Model file for the job. Use its own axes, mm. A direction names the side the tool comes from. Round coordinates to 2 decimals unless told otherwise and drop trailing zeros. Loops run counter-clockwise (first coordinate to the right, second up) from the corner with the lowest first, then second, coordinate; pieces in that order, holes last. Notation, with made-up numbers: (80, -38.75) - (119, -38.75) arc R21 ccw to (119, -14.75) - close; hole circle Ø6 at (20.25, 56). An arc over 180 degrees is marked (long way). Answer as a JSON object with one key per item and string values.
from build123d import *

# Parameters (mm, degrees)
SZKIC1_R                    = 7.5
SZKIC1_R_2                  = 5
DODANIE_WYCI_GNI_CIE1_DEPTH = 40
DODANIE_WYCI_GNI_CIE2_START = 10
SZKIC1_2_R                  = 5
DODANIE_WYCI_GNI_CIE2_DEPTH = 50
SZKIC2_OUTSIDE_W            = 29.728
SZKIC2_OUTSIDE_H            = 29.728
SZKIC2_OUTSIDE_W_2          = 10
SZKIC2_OUTSIDE_H_2          = 7
WYTNIJ_WYCI_GNI_CIE1_DEPTH  = 18
SZKIC3_R                    = 1.5
WYTNIJ_WYCI_GNI_CIE2_DEPTH  = 10


with BuildPart() as part:
    # Szkic1 → Dodanie-wyci_gni_cie1 (new body)
    with BuildSketch(Plane(origin=(0, 0, 0), x_dir=(1, 0, 0), z_dir=(0, 1, 0))):
        Circle(SZKIC1_R)
        Circle(SZKIC1_R_2, mode=Mode.SUBTRACT)
    extrude(amount=DODANIE_WYCI_GNI_CIE1_DEPTH)

    # Szkic1_2 → Dodanie-wyci_gni_cie2 (add)
    with BuildSketch(Plane(origin=(0, 0, 0), x_dir=(1, 0, 0), z_dir=(0, 1, 0)).offset(DODANIE_WYCI_GNI_CIE2_START)):
        Circle(SZKIC1_2_R)
    extrude(amount=DODANIE_WYCI_GNI_CIE2_DEPTH)

    # Szkic2 outside → Wytnij-wyci_gni_cie1 (cut)
    with BuildSketch(Plane(origin=(0, 60, 0), x_dir=(1, 0, 0), z_dir=(0, 1, 0))):
        Rectangle(SZKIC2_OUTSIDE_W, SZKIC2_OUTSIDE_H)
        Rectangle(SZKIC2_OUTSIDE_W_2, SZKIC2_OUTSIDE_H_2, mode=Mode.SUBTRACT)
    extrude(amount=-WYTNIJ_WYCI_GNI_CIE1_DEPTH, mode=Mode.SUBTRACT)

    # Szkic3 → Wytnij-wyci_gni_cie2 (cut)
    with BuildSketch(Plane.XY.offset(3.5)):
        with Locations((0, 57)):
            Circle(SZKIC3_R)
    extrude(amount=-WYTNIJ_WYCI_GNI_CIE2_DEPTH, mode=Mode.SUBTRACT)


solid = part.part
1) Two-plate mould, pull along Z, no slides. Class faces 5 (the flat face through (0, 10, 0)), 6 (the flat face through (2, 0, 5)), 7 (the flat face through (0, 51, -3.5)), 8 (the cylindrical face through (-1.08, 4.93, 4.88)): pulls with the +Z half, pulls with the -Z half, needs draft (parallel to the pull), parting line crosses it, or undercut.
Values follow:
{"face 5": "undercut", "face 6": "needs draft", "face 7": "pulls with the -Z half", "face 8": "undercut"}
2) Drop flat-ended pins along their axis: P1, Ø3, axis at x = -4.5, y = 53, coming from the +Z side; P2, Ø4, axis at x = 4, y = 28.5, coming from the +Z side; P3, Ø0.8, axis at x = 0.5, z = -4, coming from the +Y side. Give the stop position or say it passes through.
Values follow:
{"P1": "z = 3.5", "P2": "z = 7.23", "P3": "y = 42"}
3) Probe probe 1 along X at (y, z) = (2.5, 0); probe 2 along Y at (x, z) = (-4, 3.5). List the from-to ranges inside material, lowest first.
Values follow:
{"probe 1": "-7.5 to -5, 5 to 7.5", "probe 2": "0 to 40"}
4) Slice it at C-C on z = 0. List the corners of the cut face in (x, y).
Values follow:
{"outline": "(-7.5, 0) - (-5, 0) - (-5, 10) - (5, 10) - (5, 0) - (7.5, 0) - (7.5, 40) - (5, 40) - (5, 60) - (-5, 60) - (-5, 40) - (-7.5, 40) - close; hole circle Ø3 at (0, 57)"}
5) Slice it at D-D on y = 4. List the corners of the cut face in (x, z).
Values follow:
{"outline": "circle Ø15 at (0, 0); hole circle Ø10 at (0, 0)"}
6) Slice it at A-A on y = 57. List the corners of the cut face in (x, z), then the cut area to 3 significant figures.
Values follow:
{"outline": "(-3.57, -3.5) - (-1.5, -3.5) - (-1.5, 3.5) - (-3.57, 3.5) arc R5 ccw to start; (1.5, -3.5) - (3.57, -3.5) arc R5 ccw to (3.57, 3.5) - (1.5, 3.5) - close", "area": "42.8 mm²"}
7) Slice it at B-B on x = 0. List the corners of the cut face in (y, z), then the cut area to 3 significant figures.
Values follow:
{"outline": "(0, -7.5) - (40, -7.5) - (40, -5) - (42, -5) - (42, -3.5) - (55.5, -3.5) - (55.5, 3.5) - (42, 3.5) - (42, 5) - (40, 5) - (40, 7.5) - (0, 7.5) - (0, 5) - (10, 5) - (10, -5) - (0, -5) - close; (58.5, -3.5) - (60, -3.5) - (60, 3.5) - (58.5, 3.5) - close", "area": "625 mm²"}
8) Tool access for faces 1 (the cylindrical face through (-5, 50, 0)), 2 (the cylindrical face through (-0.195, 58.487, 0.049)), 3 (the flat face through (0, 51, 3.5)), 4 (the flat face through (0, 42, -4)): list every direction of +Z, -Z, +X, -X, +Y, -Y with a clear straight run to the whole face (end or side of a thin tool).
Values follow:
{"face 1": "+Y", "face 2": "+Z, -Z", "face 3": "+Z, +X, -X, +Y", "face 4": "-Z, +X, -X, +Y"}
